Input: part model. Units: mm. Frame: model coordinates. Face numbers are marked on the shaded views. A direction names the side the tool comes from. Give positions to 0.01 mm unless a question says otherwise; leave off trailing zeros. Loops run counter-clockwise (first coordinate to the right, second up) from the corner with the lowest first, then second, coordinate; pieces in that order, holes last. Notation, with made-up numbers: M 24,19.25 L 76,19.25 A12 ccw 76,27.25 Z; hole C 34,78.25 d2. An arc over 180 degrees is marked long. Answer as a JSON object with one key per item and string values. Group by question number.
1) Draft query along X for the marked faces 5, 6 and 7. Return one class per face: +X half, -X half, draft (parallel to the pull), parting line (faces both ways), or undercut.
2) Section query C-C on x = 0. Return loops of the section in (y, z).
3) First-contact query: P1, Ø1.5, axis at y = 1.5, z = 2.5, coming from the +X side; P2, Ø5, axis at y = -2, z = 7.5, coming from the +X side. Flat tips, straight axial feed; report the tip coordinate or a pass-through.
4) Section query D-D on z = 4.5. Return loops of the section in (x, y), plus the area to 3 significant figures.
5) Section query A-A on z = 8.5. Return loops of the section in (x, y), plus the area to 3 significant figures.
6) Ray query, L1, parallel to Y at x = 0, z = 3.25; L2, parallel to Z at x = -6.5, y = -2.5; L3, parallel to X at y = 1.5, z = 7.5. Return the intervals inside material, ascending.
7) Section query B-B on y = 0. Return loops of the section in (x, z).
8) Access query for the marked faces 1, 2, 3 and 4. Directions: +Z, -Z, +X, -X, +Y, -Y. A direction counts if a zero-diameter tool reaches every point of the face in a straight line with its end or side. Return the directions, or none.
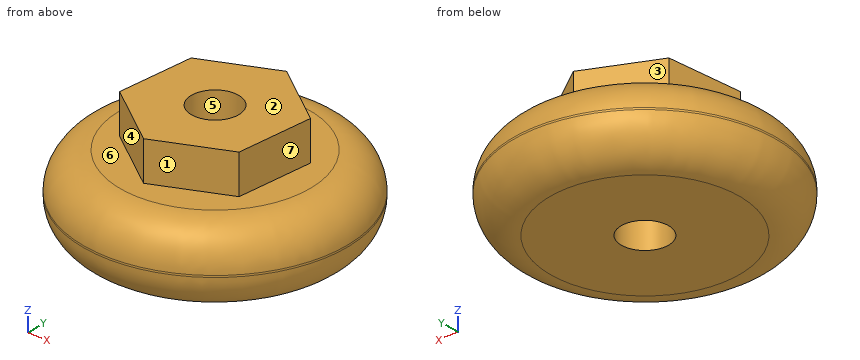
from build123d import *

# Parameters (mm, degrees)
F0_R     = 11.1125
F0_R_2   = 2
F1_DEPTH = 6.35
F2_R     = 2
F3_DEPTH = 3.3
F4_R     = 3.1


with BuildPart() as f1:
    # F0 (on Top) → F1 (new body)
    with BuildSketch(Plane.XY):
        Circle(F0_R)
        Circle(F0_R_2, mode=Mode.SUBTRACT)
    extrude(amount=F1_DEPTH)

    # F2 (on face) → F3 (join)
    with BuildSketch(Plane.XY.offset(6.35)):
        Polygon((-5.123777, 3.861277), (-5.905853, -2.506682), (-0.782076, -6.36796), (5.123777, -3.861277), (5.905853, 2.506682), (0.782076, 6.36796), align=None)
        Circle(F2_R, mode=Mode.SUBTRACT)
    extrude(amount=F3_DEPTH)

    # F4
    f4_edges = [f1.edges().sort_by_distance(p)[0] for p in [
        (-11.1125, 0, 0),
        (-11.1125, 0, 6.35),
    ]]
    fillet(f4_edges, radius=F4_R)


solid = f1.part
Output:
{
 "1": {"face 5": "undercut", "face 6": "draft", "face 7": "+X half"},
 "2": {"outline": "M -11.11,3.1 A3.1 ccw -8.01,0 L -2,0 L -2,9.65 L -6.04,9.65 L -6.04,6.35 L -8.01,6.35 A3.1 ccw -11.11,3.25 Z; M 2,0 L 8.01,0 A3.1 ccw 11.11,3.1 L 11.11,3.25 A3.1 ccw 8.01,6.35 L 6.04,6.35 L 6.04,9.65 L 2,9.65 Z"},
 "3": {"P1": "stops at x = 11.07", "P2": "stops at x = 10.43"},
 "4": {"outline": "C 0,0 d21.7; hole C 0,0 d4", "area": "357 mm^2"},
 "5": {"outline": "M -5.91,-2.51 L -0.78,-6.37 L 5.12,-3.86 L 5.91,2.51 L 0.78,6.37 L -5.12,3.86 Z; hole C 0,0 d4", "area": "94.4 mm^2"},
 "6": {"L1": "y = -11.11 to -2, 2 to 11.11", "L2": "z = 0 to 6.35", "L3": "x = -5.41 to -1.32, 1.32 to 5.78"},
 "7": {"outline": "M -11.11,3.1 A3.1 ccw -8.01,0 L -2,0 L -2,9.65 L -5.6,9.65 L -5.6,6.35 L -8.01,6.35 A3.1 ccw -11.11,3.25 Z; M 2,0 L 8.01,0 A3.1 ccw 11.11,3.1 L 11.11,3.25 A3.1 ccw 8.01,6.35 L 5.6,6.35 L 5.6,9.65 L 2,9.65 Z"},
 "8": {"face 1": "+Z, +X, -Y", "face 2": "+Z, +X, -X, +Y, -Y", "face 3": "+Z, -X, +Y", "face 4": "+Z, -X, -Y"}
}
